from build123d import *

# Parameters (mm, degrees)
SKETCH1_W           = 339.725
SKETCH1_H           = 101.6
BOSS_EXTRUDE1_DEPTH = 15.875
CUT_EXTRUDE2_START  = -15.875
SKETCH2_R           = 9.9187
CUT_EXTRUDE2_DEPTH  = 63.5
CUT_EXTRUDE4_START  = -15.875
SKETCH3_R           = 15.0876
CUT_EXTRUDE4_DEPTH  = 3.175
CUT_EXTRUDE6_START  = -15.875
SKETCH4_R           = 8.3312
CUT_EXTRUDE6_DEPTH  = 63.5


with BuildPart() as part:
    # Sketch1 → Boss-Extrude1 (new, symmetric)
    with BuildSketch(Plane(origin=(0, 0, 0), x_dir=(1, 0, 0), z_dir=(0, 1, 0))):
        Rectangle(SKETCH1_W, SKETCH1_H)
    extrude(amount=BOSS_EXTRUDE1_DEPTH, both=True)

    # Sketch2 → Cut-Extrude2 (cut)
    with BuildSketch(Plane(origin=(0, 0, 0), x_dir=(1, 0, 0), z_dir=(0, 1, 0)).offset(CUT_EXTRUDE2_START)):
        with Locations(Location((-139.7127, -12.7, 0), (0, 0, 90))):
            Circle(SKETCH2_R)
        with Locations(Location((-0.0127, -12.7, 0), (0, 0, 90))):
            Circle(SKETCH2_R)
        with Locations(Location((139.6873, -12.7, 0), (0, 0, 90))):
            Circle(SKETCH2_R)
    extrude(amount=CUT_EXTRUDE2_DEPTH, mode=Mode.SUBTRACT)

    # Sketch3 → Cut-Extrude4 (cut)
    with BuildSketch(Plane(origin=(0, 0, 0), x_dir=(1, 0, 0), z_dir=(0, 1, 0)).offset(CUT_EXTRUDE4_START)):
        with Locations(Location((-139.7127, -12.7, 0), (0, 0, 270))):
            Circle(SKETCH3_R)
        with Locations(Location((-0.0127, -12.7, 0), (0, 0, 270))):
            Circle(SKETCH3_R)
        with Locations(Location((139.6873, -12.7, 0), (0, 0, 270))):
            Circle(SKETCH3_R)
    extrude(amount=CUT_EXTRUDE4_DEPTH, mode=Mode.SUBTRACT)

    # Sketch4 → Cut-Extrude6 (cut)
    with BuildSketch(Plane(origin=(0, 0, 0), x_dir=(1, 0, 0), z_dir=(0, 1, 0)).offset(CUT_EXTRUDE6_START)):
        with Locations(Location((-88.9127, 34.925, 0), (0, 0, 90))):
            Circle(SKETCH4_R)
        with Locations(Location((88.8873, 34.925, 0), (0, 0, 90))):
            Circle(SKETCH4_R)
    extrude(amount=CUT_EXTRUDE6_DEPTH, mode=Mode.SUBTRACT)


solid = part.part
Check sheet for the modelled part. Datum: model origin and axes. Units: mm. A direction names the side the tool comes from. Round coordinates to 2 decimals unless told otherwise and drop trailing zeros. Loops run counter-clockwise (first coordinate to the right, second up) from the corner with the lowest first, then second, coordinate; pieces in that order, holes last. Notation, with made-up numbers: (64, -21) - (70, -21) arc R9 cw to (70, -8) - close; hole circle Ø7 at (33, 30.25). An arc over 180 degrees is marked (long way). Answer as CSV lines item,"result". Start each with the question number.
Item 1: Section check A-A (x = -134). Record the boundary of the cut face in (y, z) (3 decimals).
Item 2: Section check D-D (y = 11.5). Record the boundary of the cut face in (x, z) (1 decimal).
Item 3: Section check C-C (z = 12.7). Record the boundary of the cut face in (x, y) (1 decimal), and give its area (3 significant figures).
Item 4: Section check B-B (z = -33.5). Record the boundary of the cut face in (x, y) (1 decimal), and give its area (3 significant figures).
Item 5: Set-up check for faces 4 (the cylindrical face through (-2.99, 1.39, 3.24)), 5 (the flat face through (-3, -12.7, 23)): record each of +Z, -Z, +X, -X, +Y, -Y from which the full face is reachable in a straight line by a thin tool's end or side.
Item 6: Release check for a two-part mould opening along Z. For faces 1 (the flat face through (-2, 0, -50.8)), 2 (the cylindrical face through (88.52, -0.22, -26.6)), 3 (the flat face through (169.862, 0, 1)) record: +Z half, -Z half, draft (parallel to the pull), parting line (faces both ways), or undercut.
Item 7: Depth check by flat-ended pin: P1, Ø15, axis at x = -134, z = 16, coming from the -Y side. Enter the tip coordinate at first touch or a pass-through.
Item 8: Scan lines: line 1 (X direction, y = -2.75, z = 12.7); line 2 (X direction, y = 9, z = 16.5); line 3 (Y direction, x = -10, z = 18.5) (3 decimals). Record each from-to range of solid material in increasing order. Write a range as [from, to].
Report:
1,outline,"(-15.875, -50.8) - (15.875, -50.8) - (15.875, 4.592) - (-12.7, 4.592) - (-12.7, -1.264) - (-15.875, -1.264) - close; (-15.875, 26.664) - (-12.7, 26.664) - (-12.7, 20.808) - (15.875, 20.808) - (15.875, 50.8) - (-15.875, 50.8) - close"
2,outline,"(-169.9, -50.8) - (169.9, -50.8) - (169.9, 50.8) - (-169.9, 50.8) - close; hole circle Ø19.8 at (-139.7, 12.7); hole circle Ø16.7 at (-88.9, -34.9); hole circle Ø19.8 at (0, 12.7); hole circle Ø16.7 at (88.9, -34.9); hole circle Ø19.8 at (139.7, 12.7)"
3,outline,"(-169.9, -15.9) - (-154.8, -15.9) - (-154.8, -12.7) - (-149.6, -12.7) - (-149.6, 15.9) - (-169.9, 15.9) - close; (-129.8, -12.7) - (-124.6, -12.7) - (-124.6, -15.9) - (-15.1, -15.9) - (-15.1, -12.7) - (-9.9, -12.7) - (-9.9, 15.9) - (-129.8, 15.9) - close; (9.9, -12.7) - (15.1, -12.7) - (15.1, -15.9) - (124.6, -15.9) - (124.6, -12.7) - (129.8, -12.7) - (129.8, 15.9) - (9.9, 15.9) - close; (149.6, -12.7) - (154.8, -12.7) - (154.8, -15.9) - (169.9, -15.9) - (169.9, 15.9) - (149.6, 15.9) - close"
3,area,"8,800 mm2"
4,outline,"(-169.9, -15.9) - (-97.1, -15.9) - (-97.1, 15.9) - (-169.9, 15.9) - close; (-80.7, -15.9) - (80.7, -15.9) - (80.7, 15.9) - (-80.7, 15.9) - close; (97.1, -15.9) - (169.9, -15.9) - (169.9, 15.9) - (97.1, 15.9) - close"
4,area,"9,740 mm2"
5,face 4,"+Y, -Y"
5,face 5,"-Y"
6,face 1,"-Z half"
6,face 2,"undercut"
6,face 3,"draft"
7,P1,"stops at y = -12.7"
8,line 1,"x = [-169.86, -149.63], [-129.79, -9.93], [9.91, 129.77], [149.61, 169.86]"
8,line 2,"x = [-169.86, -148.87], [-130.55, -9.17], [9.15, 130.53], [148.85, 169.86]"
8,line 3,"y = [-12.7, 15.875]"
